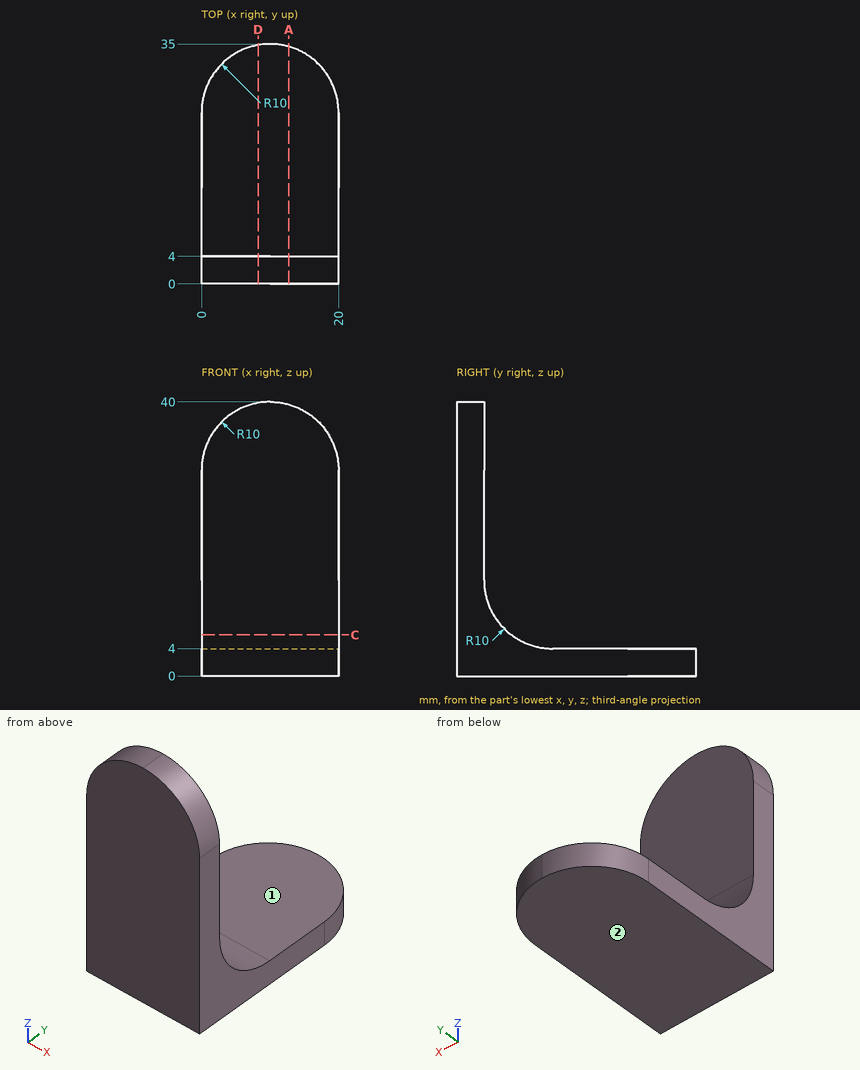
For this review, use the dimensioned drawing (mm, ordinates from the lowest corner) and the shaded views. A direction names the side the tool comes from. Coordinates: 2 decimals unless noted, no trailing zeros. Loops run counter-clockwise (first coordinate to the right, second up) from the corner with the lowest first, then second, coordinate; pieces in that order, holes last.
1. Add section C-C, the plane z = 6. Give the boundary of the cut face in (x, y), then the cut area to 3 significant figures.
2. Add section A-A, the plane x = 12.75. Give the boundary of the cut face in (y, z).
3. Add section D-D, the plane x = 8.25. Give the boundary of the cut face in (y, z), then the cut area to 3 significant figures.
4. For the marked faces 1 and 2, list the 3-axis set-ups (+Z, -Z, +X, -X, +Y, -Y) from which the entire face can be reached by the end or side of a thin tool; tool diameter is ignored.
5. For line 1 (Y direction, x = 16.5, z = 15); line 2 (Y direction, x = 15.75, z = 6.5), list the stretches that pass through material, from the lowest coordinate up.
6. Insertion check: P1, Ø5, axis at x = 11.5, y = 8.5, coming from the +Z side; P2, Ø10, axis at x = 10.5, y = 26, coming from the +Z side; P3, Ø6, axis at x = 15, z = 31.5, coming from the +Y side. Each pin has a flat end and moves straight along its axis. Give the tip position at first contact, or say it passes through.
Result:
1. outline: (0, 0) - (20, 0) - (20, 8) - (0, 8) - close
1. area: 160 mm2
2. outline: (0, 0) - (34.61, 0) - (34.61, 4) - (14, 4) arc R10 cw to (4, 14) - (4, 39.61) - (0, 39.61) - close
3. outline: (0, 0) - (34.85, 0) - (34.85, 4) - (14, 4) arc R10 cw to (4, 14) - (4, 39.85) - (0, 39.85) - close
3. area: 304 mm2
4. face 1: +Z, +X, -X, +Y
4. face 2: -Z, +X, -X, +Y, -Y
5. line 1: y = 0 to 4
5. line 2: y = 0 to 7.39
6. P1: stops at z = 8
6. P2: stops at z = 4
6. P3: stops at y = 4
